Verification items for the finished model (mm, model axes). Face numbers are marked on the shaded views. A direction names the side the tool comes from. Give positions to 0.01 mm unless a question says otherwise; leave off trailing zeros. Order: outer loops, then holes, each group sorted by start corner. A loop starts at its lowest first (then second) coordinate and runs counter-clockwise, first axis right, second up. Notation, with made-up numbers: (62.5, 7.5) - (76.5, 7.5) arc R7 ccw to (76.5, 17.5) - close; hole circle Ø10 at (44, -3). An arc over 180 degrees is marked (long way). Answer as a JSON object with one key per item and string values.
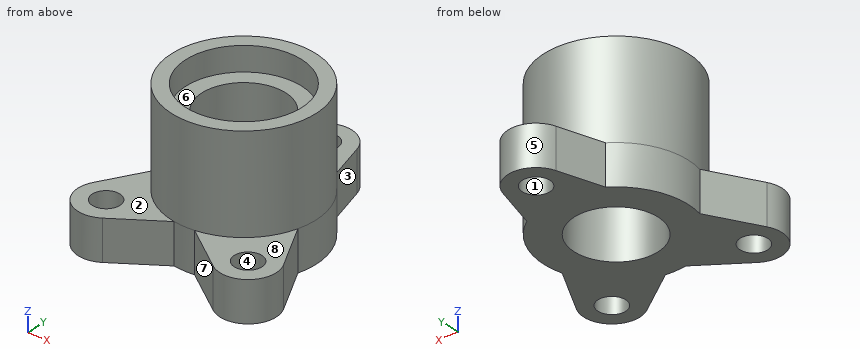
```python
from build123d import *
from build123d.topology import SkipClean

# Parameters (mm, degrees)
SKETCH1_R           = 5.225
SKETCH1_R_2         = 1.725
BOSS_EXTRUDE1_DEPTH = 5
SKETCH2_R           = 9
SKETCH2_R_2         = 5.225
BOSS_EXTRUDE2_DEPTH = 12
CUT_EXTRUDE1_START  = -3
SKETCH3_R           = 7.225
SKETCH3_R_2         = 5.225
CUT_EXTRUDE1_DEPTH  = 3


with BuildPart() as part:
    # Sketch1 → Boss-Extrude1 (new body)
    with BuildSketch(Plane.XY):
        with BuildLine():
            Line((8.72254439, -2.217480408), (12.068556171, -8.316562141))
            ThreePointArc((12.068556171, -8.316562141), (11.341376561, -12.601529512), (7.003749271, -12.87488835))
            Line((7.003749271, -12.87488835), (1.289602928, -8.907127724))
            ThreePointArc((1.289602928, -8.907127724), (0, -9), (-1.289602928, -8.907127724))
            Line((-1.289602928, -8.907127724), (-7.003749271, -12.87488835))
            ThreePointArc((-7.003749271, -12.87488835), (-11.341376561, -12.601529512), (-12.068556171, -8.316562141))
            Line((-12.068556171, -8.316562141), (-8.72254439, -2.217480408))
            ThreePointArc((-8.72254439, -2.217480408), (-8.402583705, 3.224373905), (-5, 7.483314774))
            Line((-5, 7.483314774), (-3.353912105, 13.000636594))
            ThreePointArc((-3.353912105, 13.000636594), (0, 15.5), (3.353912105, 13.000636594))
            Line((3.353912105, 13.000636594), (5, 7.483314774))
            ThreePointArc((5, 7.483314774), (8.402583705, 3.224373905), (8.72254439, -2.217480408))
        make_face()
        Circle(SKETCH1_R, mode=Mode.SUBTRACT)
        with Locations((9, -10)):
            Circle(SKETCH1_R_2, mode=Mode.SUBTRACT)
        with Locations(Location((-9, -10, 0), (0, 0, 180))):
            Circle(SKETCH1_R_2, mode=Mode.SUBTRACT)
        with Locations((0, 12)):
            Circle(SKETCH1_R_2, mode=Mode.SUBTRACT)
    extrude(amount=BOSS_EXTRUDE1_DEPTH)

    # Sketch2 → Boss-Extrude2 (add)
    with SkipClean():  # the faces are left unmerged after this step: merging them gives an invalid solid
        with BuildSketch(Plane.XY.offset(5)):
            with Locations(Location((0, 0, 0), (0, 0, 194.263798908))):
                Circle(SKETCH2_R)
            Circle(SKETCH2_R_2, mode=Mode.SUBTRACT)
        extrude(amount=BOSS_EXTRUDE2_DEPTH)

    # Sketch3 → Cut-Extrude1 (cut)
    with SkipClean():  # the faces are left unmerged after this step: merging them gives an invalid solid
        with BuildSketch(Plane.XY.offset(17).offset(CUT_EXTRUDE1_START)):
            Circle(SKETCH3_R)
            Circle(SKETCH3_R_2, mode=Mode.SUBTRACT)
        extrude(amount=CUT_EXTRUDE1_DEPTH, mode=Mode.SUBTRACT)


solid = part.part
```
(1) Section check D-D (x = 10.25). Record the cut outline in (y, z).
Computed values:
{"outline": "(-13.27, 0) - (-11.19, 0) - (-11.19, 5) - (-13.27, 5) - close; (-8.81, 0) - (-5, 0) - (-5, 5) - (-8.81, 5) - close"}
(2) Section check A-A (y = 0). Record the cut outline in (x, z) (3 decimals).
Computed values:
{"outline": "(-9, 0) - (-5.225, 0) - (-5.225, 14) - (-7.225, 14) - (-7.225, 17) - (-9, 17) - close; (5.225, 0) - (9, 0) - (9, 17) - (7.225, 17) - (7.225, 14) - (5.225, 14) - close"}
(3) Access from +Z, -Z, +X, -X, +Y, -Y to the whole of each face (thin tool, end or side, straight path). Record for the marked faces 4, 5, 6, 7 and 8.
Computed values:
{"face 4": "+Z, -Z", "face 5": "+Z, -Z, +Y", "face 6": "+Z", "face 7": "+Z, -Z, -Y", "face 8": "+Z, +X, -Y"}
(4) Section check C-C (x = 0). Record the cut outline in (y, z) (3 decimals).
Computed values:
{"outline": "(-9, 0) - (-5.225, 0) - (-5.225, 14) - (-7.225, 14) - (-7.225, 17) - (-9, 17) - close; (5.225, 0) - (10.275, 0) - (10.275, 5) - (9, 5) - (9, 17) - (7.225, 17) - (7.225, 14) - (5.225, 14) - close; (13.725, 0) - (15.5, 0) - (15.5, 5) - (13.725, 5) - close"}
(5) Material ranges on line 1 along Y through (x, z) = (0, 16.4) (3 decimals); line 2 along X through (y, z) = (0.25, 1.5); line 3 along X through (y, z) = (-4, 11.25), recorded low to high. Write a range as [from, to].
Computed values:
{"line 1": "y = [-9, -7.225], [7.225, 9]", "line 2": "x = [-9, -5.22], [5.22, 9]", "line 3": "x = [-8.06, -3.36], [3.36, 8.06]"}
(6) Release check for a two-part mould opening along X. For the marked faces 1, 2 and 3 record: pulls with the +X half, pulls with the -X half, needs draft (parallel to the pull), parting line crosses it, or undercut.
Computed values:
{"face 1": "undercut", "face 2": "needs draft", "face 3": "pulls with the +X half"}
(7) Section check B-B (z = 2.25). Record the cut outline in (x, y) (3 decimals), then the cut area to 3 significant figures.
Computed values:
{"outline": "(-12.069, -8.317) arc R3.5 ccw to (-7.004, -12.875) - (-1.29, -8.907) arc R9 ccw to (1.29, -8.907) - (7.004, -12.875) arc R3.5 ccw to (12.069, -8.317) - (8.723, -2.217) arc R9 ccw to (5, 7.483) - (3.354, 13.001) arc R3.5 ccw to (-3.354, 13.001) - (-5, 7.483) arc R9 ccw to (-8.723, -2.217) - close; hole circle Ø3.45 at (-9, -10); hole circle Ø10.45 at (0, 0); hole circle Ø3.45 at (0, 12); hole circle Ø3.45 at (9, -10)", "area": "309 mm²"}
(8) Gauge pin test, flat ends, axial feed: pin 1 Ø6 at (x, z) = (-4.5, 2) entering from -Y; pin 2 Ø10 at (y, z) = (11, 10) entering from +X; pin 3 Ø2.5 at (x, y) = (1.5, 12) entering from +Z; pin 4 Ø4 at (x, y) = (-2, 1.5) entering from +Z. Record the tip position at first contact, or that the pin passes through.
Computed values:
{"pin 1": "stops at y = -13.16", "pin 2": "stops at x = 6.71", "pin 3": "stops at z = 5", "pin 4": "passes through"}
